Input: dimensioned drawing with shaded views. Units: mm. Origin: part minimum x, y, z. A direction names the side the tool comes from. Round coordinates to 2 decimals unless told otherwise and drop trailing zeros. Order: outer loops, then holes, each group sorted by start corner. A loop starts at its lowest first (then second) coordinate and runs counter-clockwise, first axis right, second up. Notation, with made-up numbers: (-20.5, -24.75) - (13.5, -24.75) arc R24 cw to (13.5, 9.25) - close; hole circle Ø6 at (9.5, -24). An arc over 180 degrees is marked (long way). Put each result on its own line as item: value. Start each with the question number.
(1) Pin query (flat end, axial travel): P1, Ø3, axis at x = 201.5, z = 29.5, coming from the -Y side; P2, Ø4.5, axis at x = 139.7, y = 12.7, coming from the -Z side. Return the tip coordinate at first contact, or that it passes through.
(2) Section D-D (y = 88.9). Count the separate pieces of the cut face and the enclosed holes in it, and give its area (3 significant figures).
(3) Section B-B (z = 22.5). Output: boundary loops of the cut face in (x, y), and give its area (3 significant figures).
(4) Access query for the marked faces 1 and 2. Directions: +Z, -Z, +X, -X, +Y, -Y. A direction counts if a zero-diameter tool reaches every point of the face in a straight line with its end or side. Return the directions, or none.
(5) Material intervals for L1, parallel to Y at x = 190.5, z = 49.9; L2, parallel to Y at x = 114, z = 50 (1 decimal); L3, parallel to Z at x = 76, y = 16, sorted ascending. Write a range as [from, to].
(6) Section C-C (x = 27). Output: boundary loops of the cut face in (y, z).
(7) Pull-direction query (Z, two-part tool) for the marked faces 3, 4 and 5; classes: released by +Z, released by -Z, zero draft, split by the parting line, or undercut.
(8) Section A-A (y = 50.5). Output: boundary loops of the cut face in (x, z).
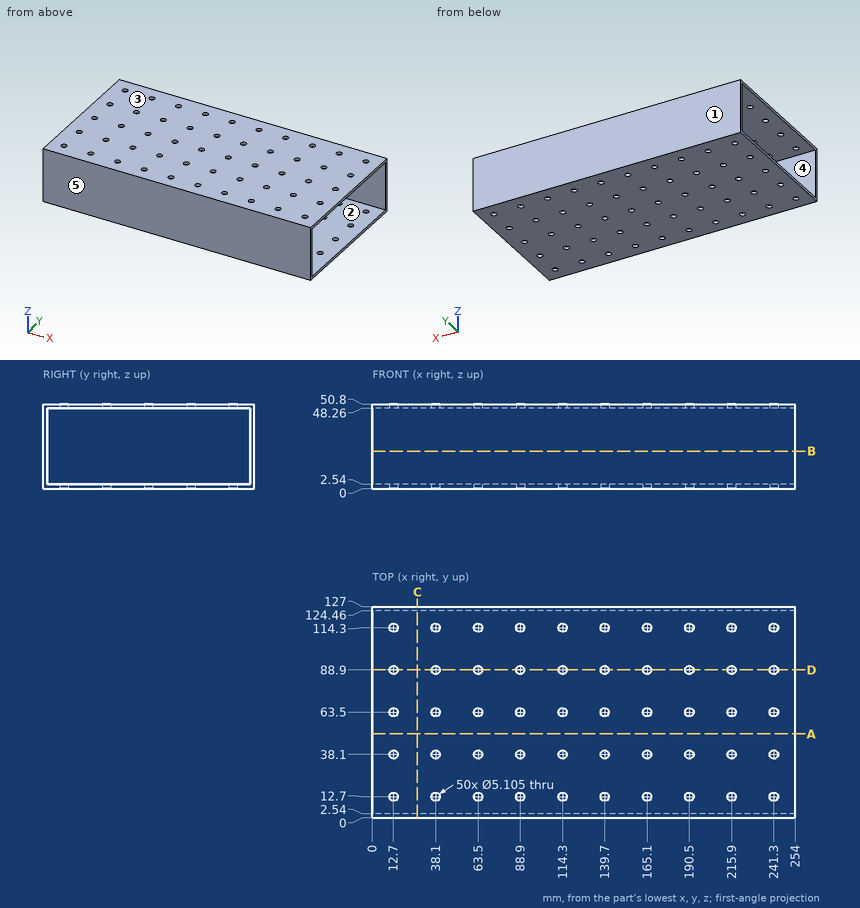
Checks:
1. P1: stops at y = 0
1. P2: passes through
2. separate pieces: 22
2. enclosed holes: 0
2. area: 1,030 mm²
3. outline: (0, 0) - (254, 0) - (254, 2.54) - (0, 2.54) - close; (0, 124.46) - (254, 124.46) - (254, 127) - (0, 127) - close
3. area: 1,290 mm²
4. face 1: +Z, -Z, +X, -X, +Y
4. face 2: +X, -X
5. L1: y = [0, 10.15], [15.25, 35.55], [40.65, 60.95], [66.05, 86.35], [91.45, 111.75], [116.85, 127]
5. L2: y = [0, 10.2], [15.2, 35.6], [40.6, 61], [66, 86.4], [91.4, 111.8], [116.8, 127]
5. L3: z = [0, 2.54], [48.26, 50.8]
6. outline: (0, 0) - (127, 0) - (127, 50.8) - (0, 50.8) - close; hole (2.54, 2.54) - (124.46, 2.54) - (124.46, 48.26) - (2.54, 48.26) - close
7. face 3: released by +Z
7. face 4: undercut
7. face 5: zero draft
8. outline: (0, 0) - (254, 0) - (254, 2.54) - (0, 2.54) - close; (0, 48.26) - (254, 48.26) - (254, 50.8) - (0, 50.8) - close
